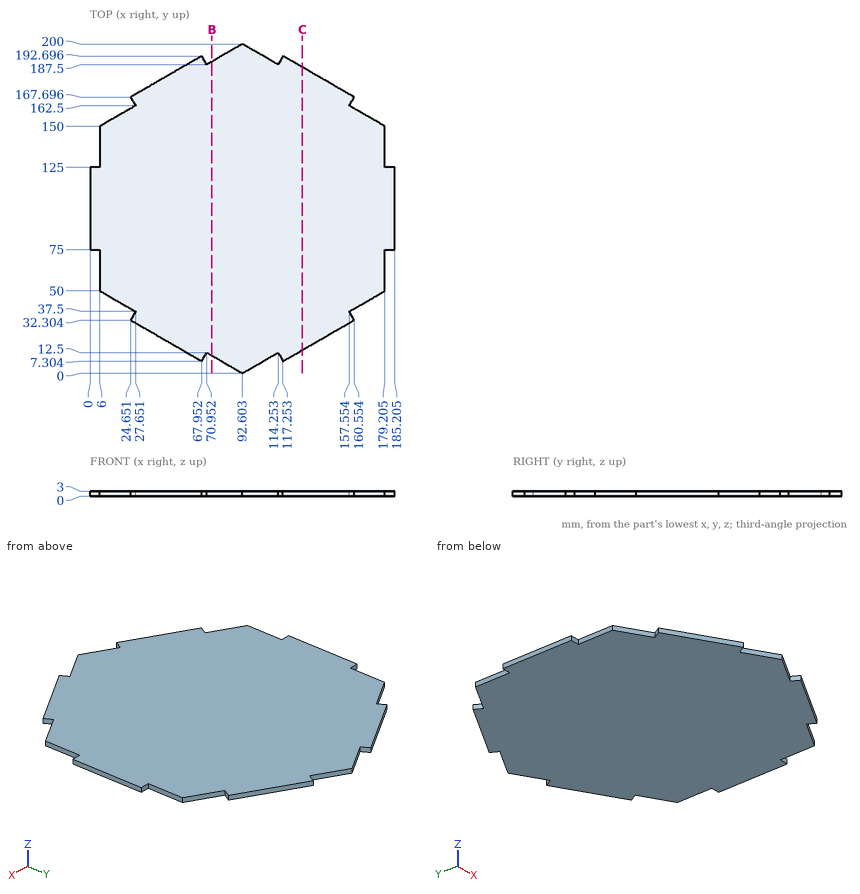
Geometry check sheet. Reference: drawing and pictorial views, mm from the part's lowest x, y, z. Round coordinates to 2 decimals unless told otherwise and drop trailing zeros. Write each loop counter-clockwise with the first axis right and the second up, starting at its lowest first coordinate (ties: lowest second). Pieces come first, ordered by that corner, then holes. Notation, with made-up numbers: (-1.75, 88.25) -> (23.25, 88.25) arc R9 cw to (23.25, 99.25) -> close; hole circle Ø9 at (-31, 67). An arc over 180 degrees is marked (long way). One line per question, with ' | ' between items. Start each with the question number.
1. Sectioned sample at B-B, the plane x = 74. Record the cut outline in (y, z).
2. Depth check by flat-ended pin: pin 1 (1.5 mm diameter, centred on y = 136, z = 1, fed in from +X) (1 decimal); pin 2 (1.5 mm diameter, centred on x = 43, z = 1, fed in from -Y); pin 3 (1.5 mm diameter, centred on x = 3, z = 2, fed in from -Y). Enter the tip coordinate at first touch or a pass-through.
3. Scan lines: line 1 along Y through (x, z) = (59, 0.8); line 2 along X through (y, z) = (146, 1.3) (1 decimal); line 3 along Y through (x, z) = (34, 2.7) (1 decimal). Record each from-to range of solid material in increasing order. Write a range as from..to.
4. Sectioned sample at C-C, the plane x = 129. Record the cut outline in (y, z) (1 decimal).
Taken from the geometry:
1) outline: (10.74, 0) -> (189.26, 0) -> (189.26, 3) -> (10.74, 3) -> close
2) pin 1: stops at x = 179.2 | pin 2: stops at y = 21.28 | pin 3: stops at y = 75
3) line 1: y = 12.47..187.53 | line 2: x = 6..179.2 | line 3: y = 26.9..173.1
4) outline: (14.1, 0) -> (185.9, 0) -> (185.9, 3) -> (14.1, 3) -> close
